The figure shows three views and two pictorial views of one solid part (mm, origin at its lowest corner). Answer the questions. A direction names the side the tool comes from. Round coordinates to 2 decimals unless told otherwise and drop trailing zeros. Loops run counter-clockwise (first coordinate to the right, second up) from the corner with the lowest first, then second, coordinate; pieces in that order, holes last. Notation, with made-up numbers: (62, 46) -> (106, 46) arc R7 cw to (106, 56) -> close; hole circle Ø5 at (-36.75, 54). An arc over 180 degrees is marked (long way). Use a Markdown table: item, result. Add a question column.
Q1. Given pin 1 Ø8 at (x, y) = (33, 14) entering from +Z; pin 2 Ø10 at (x, y) = (49, 46) entering from +Z; pin 3 Ø3 at (x, z) = (66, 56) entering from -Y, each flat-ended and moving along its own axis, determine where each tip first touches the part or whether it passes through.
Q2. Consider line 1 (Y direction, x = 61.5, z = 5.5); line 2 (X direction, y = 23.5, z = 36.5); line 3 (X direction, y = 32.5, z = 10). Determine where each line is inside the solid, lowest interval first.
Q3. Section A-A on y = 13.5 is taken. Give the vertices of the cut face in (x, z).
Q4. Section B-B on z = 54 is taken. Give the vertices of the cut face in (x, y), then the cut area to 3 significant figures.
Q5. Section C-C on x = 6 is taken. Give the vertices of the cut face in (y, z).
Q6. Which of the six approach directions +Z, -Z, +X, -X, +Y, -Y give full straight-line access (tool end or side, diameter ignored) to the marked faces 1, 2 and 3?
Q7. Section D-D on z = 6.5 is taken. Give the vertices of the cut face in (x, y).
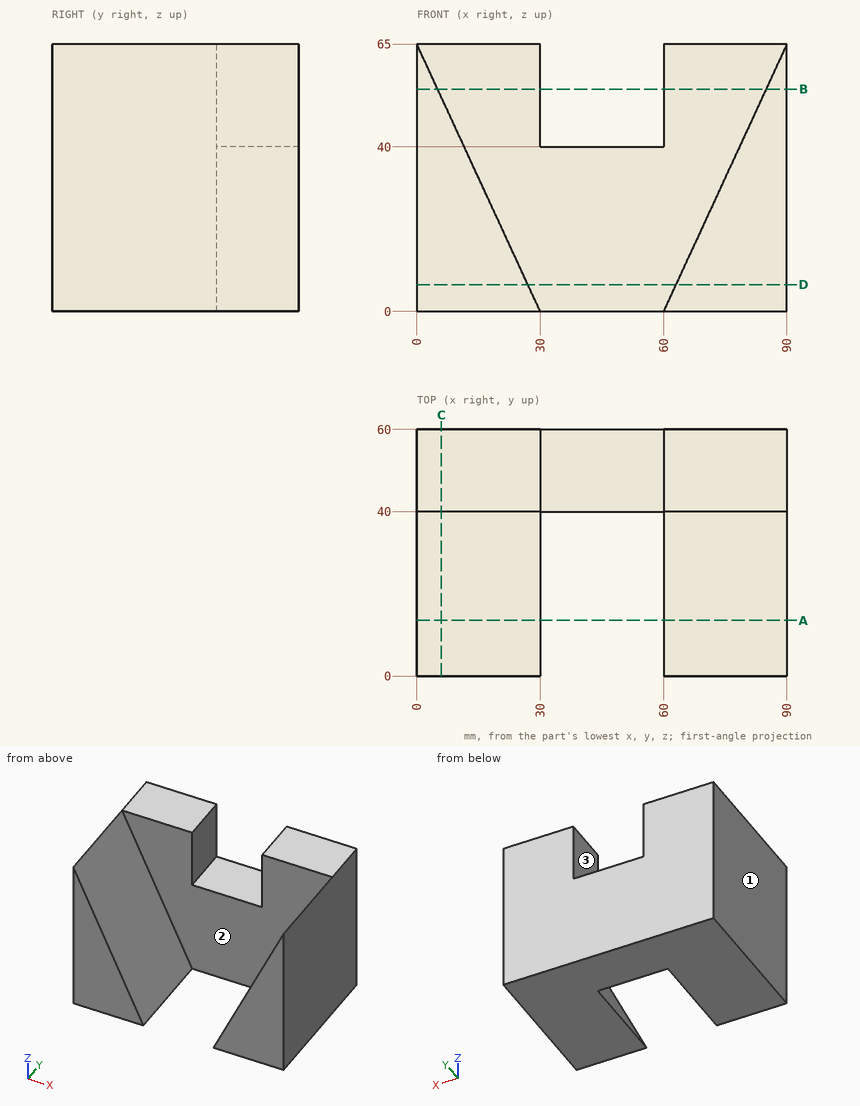
Checked values:
| question | item | result |
|---|---|---|
| 1 | pin 1 | stops at z = 2.17 |
| 1 | pin 2 | stops at z = 40 |
| 1 | pin 3 | stops at y = 40 |
| 2 | line 1 | y = 40 to 60 |
| 2 | line 2 | x = 0 to 13.15, 76.85 to 90 |
| 2 | line 3 | x = 0 to 25.38, 64.62 to 90 |
| 3 | outline | (0, 0) -> (30, 0) -> (0, 65) -> close; (60, 0) -> (90, 0) -> (90, 65) -> close |
| 4 | outline | (0, 0) -> (5.08, 0) -> (5.08, 40) -> (30, 40) -> (30, 60) -> (0, 60) -> close; (60, 40) -> (84.92, 40) -> (84.92, 0) -> (90, 0) -> (90, 60) -> (60, 60) -> close |
| 4 | area | 1,610 mm2 |
| 5 | outline | (0, 0) -> (60, 0) -> (60, 65) -> (40, 65) -> (40, 52) -> (0, 52) -> close |
| 6 | face 1 | +Z, -Z, -X, +Y, -Y |
| 6 | face 2 | +Z, -Y |
| 6 | face 3 | +Z, +Y, -Y |
| 7 | outline | (0, 0) -> (27, 0) -> (27, 40) -> (63, 40) -> (63, 0) -> (90, 0) -> (90, 60) -> (0, 60) -> close |
